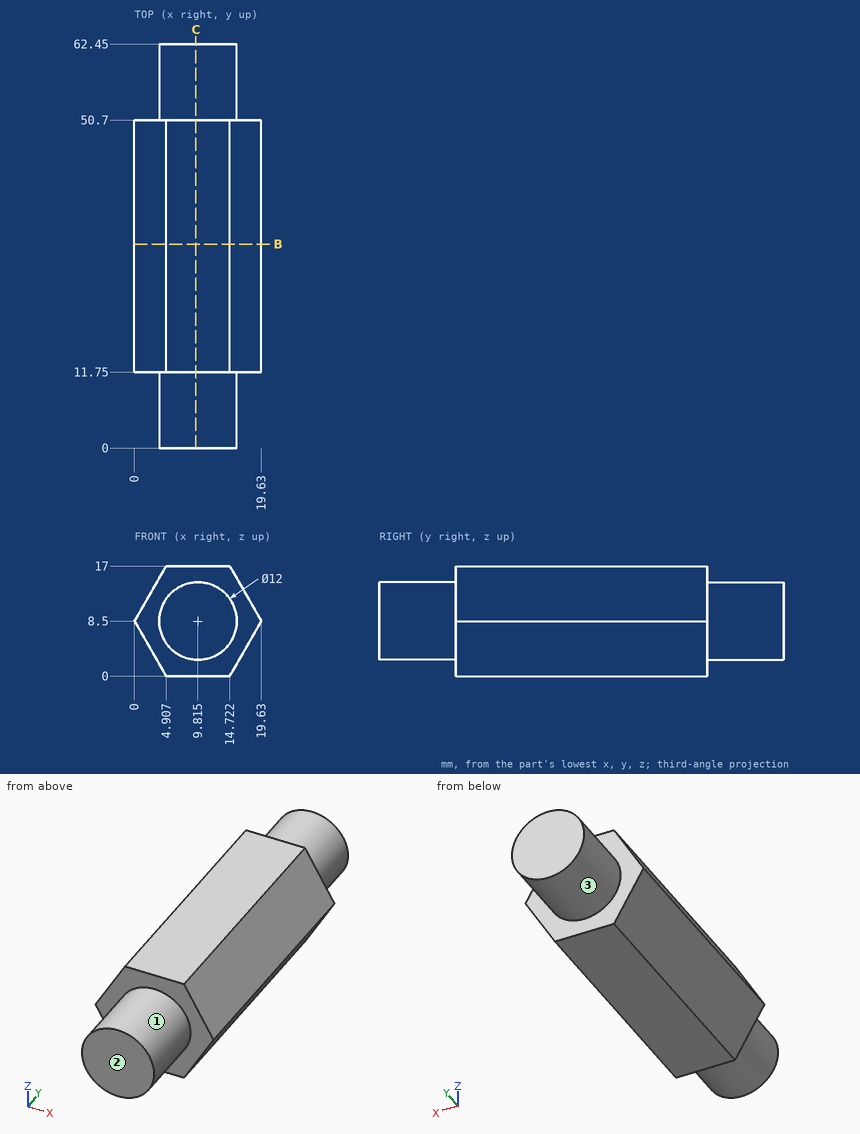
For this review, use the dimensioned drawing (mm, ordinates from the lowest corner) and the shaded views. A direction names the side the tool comes from. Coordinates: 2 decimals unless noted, no trailing zeros. Loops run counter-clockwise (first coordinate to the right, second up) from the corner with the lowest first, then second, coordinate; pieces in that order, holes last.
1. Add section B-B, the plane y = 31.5. Give the boundary of the cut face in (x, z), then the cut area to 3 significant figures.
2. For line 1 (Y direction, x = 17.25, z = 5.5); line 2 (X direction, y = 43, z = 13.75); line 3 (Z direction, x = 2.5, y = 17), list the stretches that pass through material, from the lowest coordinate up.
3. Insertion check: P1, Ø1.5, axis at y = 11.5, z = 13, coming from the -X side; P2, Ø1.5, axis at y = 27.5, z = 12, coming from the +X side; P3, Ø1, axis at x = 7, y = 53, coming from the +Z side (1 decimal). Each pin has a flat end and moves straight along its axis. Give the tip position at first contact, or say it passes through.
4. Add section C-C, the plane x = 9.5. Give the boundary of the cut face in (y, z).
5. For the marked faces 1, 2 and 3, list the 3-axis set-ups (+Z, -Z, +X, -X, +Y, -Y) from which the entire face can be reached by the end or side of a thin tool; tool diameter is ignored.
Result:
1. outline: (0, 8.5) - (4.91, 0) - (14.72, 0) - (19.63, 8.5) - (14.72, 17) - (4.91, 17) - close
1. area: 250 mm2
2. line 1: y = 11.75 to 50.7
2. line 2: x = 3.03 to 16.6
2. line 3: z = 4.17 to 12.83
3. P1: stops at x = 2.19
3. P2: stops at x = 18.04
3. P3: stops at z = 14
4. outline: (0, 2.51) - (11.75, 2.51) - (11.75, 0) - (50.7, 0) - (50.7, 2.51) - (62.45, 2.51) - (62.45, 14.49) - (50.7, 14.49) - (50.7, 17) - (11.75, 17) - (11.75, 14.49) - (0, 14.49) - close
5. face 1: -Y
5. face 2: +Z, -Z, +X, -X, -Y
5. face 3: +Y
